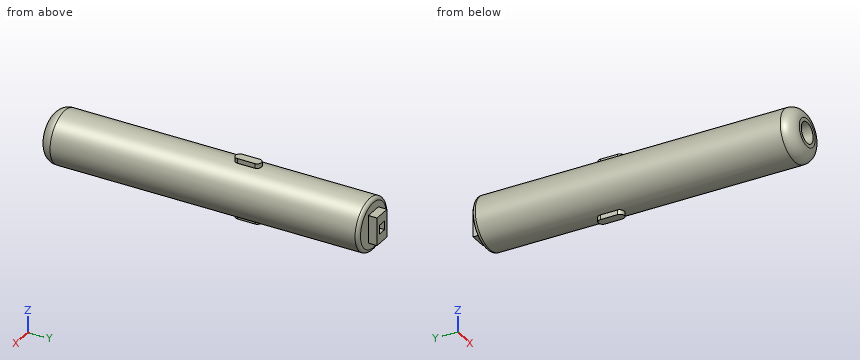
from build123d import *

# Parameters (mm, degrees)
SKETCH1_R                = 15
BOSS_EXTRUDE1_DEPTH      = 185
FILLET2_R                = 7
FILLET3_R                = 2
SKETCH2_R                = 6
CUT_EXTRUDE1_DEPTH       = 180
BOSS_EXTRUDE3_DEPTH      = 2.5
BOSS_EXTRUDE3_DEPTH_BACK = 32.5
BOSS_EXTRUDE4_START      = 185
BOSS_EXTRUDE4_DEPTH      = 5
CUT_EXTRUDE3_DEPTH       = 3


with BuildPart() as part:
    # Sketch1 → Boss-Extrude1 (new body)
    with BuildSketch(Plane(origin=(0, 0, 0), x_dir=(1, 0, 0), z_dir=(0, 1, 0))):
        Circle(SKETCH1_R)
    extrude(amount=BOSS_EXTRUDE1_DEPTH)

    # Fillet2
    fillet2_edges = [part.edges().sort_by_distance(p)[0] for p in [
        (-15, 0, 0),
    ]]
    fillet(fillet2_edges, radius=FILLET2_R)

    # Fillet3
    fillet3_edges = [part.edges().sort_by_distance(p)[0] for p in [
        (-15, 185, 0),
    ]]
    fillet(fillet3_edges, radius=FILLET3_R)

    # Sketch2 → Cut-Extrude1 (cut)
    with BuildSketch(Plane(origin=(0, 0, 0), x_dir=(1, 0, 0), z_dir=(0, 1, 0))):
        Circle(SKETCH2_R)
    extrude(amount=CUT_EXTRUDE1_DEPTH, mode=Mode.SUBTRACT)

    # Sketch7 → Boss-Extrude3 (add, two sides)
    with BuildSketch(Plane.XY.offset(15)) as boss_extrude3_sk:
        with BuildLine():
            Line((2.5, 113), (2.5, 118))
            ThreePointArc((2.5, 118), (0, 120.5), (-2.5, 118))
            Line((-2.5, 118), (-2.5, 113))
            Line((-2.5, 113), (-2.5, 108))
            ThreePointArc((-2.5, 108), (0, 105.5), (2.5, 108))
            Line((2.5, 108), (2.5, 113))
        make_face()
    extrude(amount=BOSS_EXTRUDE3_DEPTH)
    extrude(boss_extrude3_sk.sketch, amount=-BOSS_EXTRUDE3_DEPTH_BACK)

    # Sketch8 → Boss-Extrude4 (add)
    with BuildSketch(Plane(origin=(0, 0, 0), x_dir=(1, 0, 0), z_dir=(0, 1, 0)).offset(BOSS_EXTRUDE4_START)):
        Polygon((0, 8), (-5, 8), (-5, 0), (-5, -8), (0, -8), (5, -8), (5, 0), (5, 8), align=None)
    extrude(amount=BOSS_EXTRUDE4_DEPTH)

    # Sketch10 → Cut-Extrude3 (cut)
    with BuildSketch(Plane(origin=(0, 190, 0), x_dir=(1, 0, 0), z_dir=(0, 1, 0))):
        Polygon((0, -2.5), (2.5, -2.5), (2.5, 2.5), (0, 2.5), (-2.5, 2.5), (-2.5, -2.5), align=None)
    extrude(amount=-CUT_EXTRUDE3_DEPTH, mode=Mode.SUBTRACT)


solid = part.part
Design review of the part built by this model. Coordinates are the model's own, in mm. Give positions to 0.01 mm unless a question says otherwise; leave off trailing zeros. Loops run counter-clockwise (first coordinate to the right, second up) from the corner with the lowest first, then second, coordinate; pieces in that order, holes last. Notation, with made-up numbers: M 77,28.5 L 114,28.5 A18 cw 114,32.5 Z; hole C 17.25,46 d5. An arc over 180 degrees is marked long. One line per question, with ' | ' between items. Start each with the question number.
1. To check wall thickness, follow L1, parallel to X at y = 108, z = 0; L2, parallel to X at y = 129, z = 0; L3, parallel to X at y = 119, z = -1.5. State the ranges of each line that lie inside material, in increasing order.
2. Insertion check: P1, Ø0.9, axis at y = 188.5, z = -0.5, coming from the +X side; P2, Ø2, axis at y = 114.5, z = -16.5, coming from the +X side; P3, Ø1, axis at x = 6, z = 0.5, coming from the +Y side; P4, Ø4, axis at x = 0.5, z = 1, coming from the +Y side. Each pin has a flat end and moves straight along its axis. Give the tip position at first contact, or say it passes through.
3. Add section B-B (z = 0). Write out the cut boundary in (x, y), plus the area to 3 significant figures.
4. Add section C-C (y = 168). Write out the cut boundary in (x, z).
Worked out:
1) L1: x = -15 to -6, -2.5 to 2.5, 6 to 15 | L2: x = -15 to -6, 6 to 15 | L3: x = -14.92 to -5.81, -2.29 to 2.29, 5.81 to 14.92
2) P1: stops at x = 5 | P2: stops at x = 2.5 | P3: stops at y = 185 | P4: stops at y = 190
3) outline: M -15,7 A7 ccw -8,0 L -6,0 L -6,180 L 6,180 L 6,0 L 8,0 A7 ccw 15,7 L 15,183 A2 ccw 13,185 L 5,185 L 5,190 L 2.5,190 L 2.5,187 L -2.5,187 L -2.5,190 L -5,190 L -5,185 L -13,185 A2 ccw -15,183 Z; M -2.5,108 A2.5 ccw 2.5,108 L 2.5,118 A2.5 ccw -2.5,118 Z | area: 3,470 mm²
4) outline: C 0,0 d30; hole C 0,0 d12
